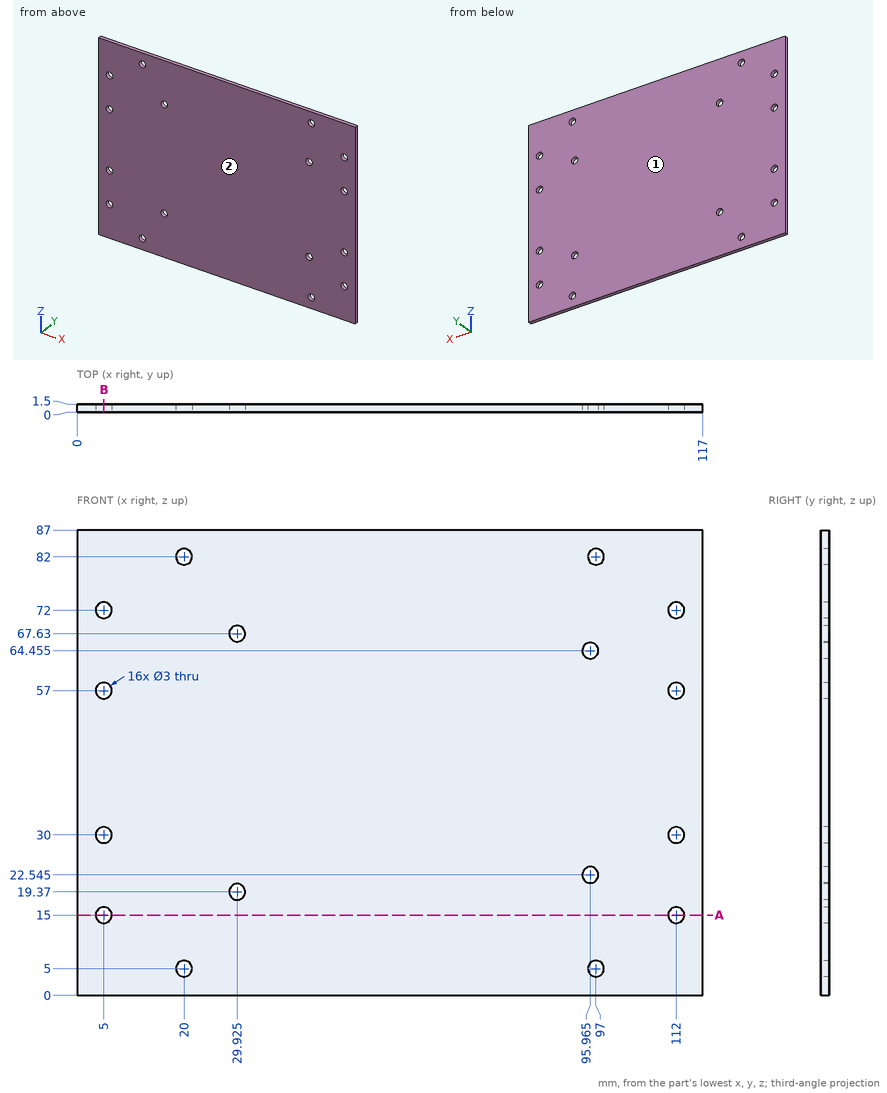
The figure shows three views and two pictorial views of one solid part (mm, origin at its lowest corner). Answer the questions. Give positions to 0.01 mm unless a question says otherwise; leave off trailing zeros. Order: outer loops, then holes, each group sorted by start corner. A loop starts at its lowest first (then second) coordinate and runs counter-clockwise, first axis right, second up. Notation, with made-up numbers: (81, -35) -> (116, -35) arc R8 ccw to (116, -28) -> close; hole circle Ø2 at (15.5, -4). An arc over 180 degrees is marked (long way). One line per item, written item: value.
1) Find the intervals of material crossed by line 1 (Z direction, x = 20, y = 1.2); line 2 (Z direction, x = 112, y = 0.75); line 3 (X direction, y = 0.55, z = 82), in increasing order.
Reported:
line 1: z = 0 to 3.5, 6.5 to 80.5, 83.5 to 87
line 2: z = 0 to 13.5, 16.5 to 28.5, 31.5 to 55.5, 58.5 to 70.5, 73.5 to 87
line 3: x = 0 to 18.5, 21.5 to 95.5, 98.5 to 117
2) Determine the mould class of the marked faces 1 and 2 for opening direction Y: pulls with the +Y half, pulls with the -Y half, needs draft (parallel to the pull), parting line crosses it, or undercut.
Reported:
face 1: pulls with the +Y half
face 2: pulls with the -Y half
3) Find section B-B, the plane x = 5. Determine the outline of the cut face in (y, z).
Reported:
outline: (0, 0) -> (1.5, 0) -> (1.5, 13.5) -> (0, 13.5) -> close; (0, 16.5) -> (1.5, 16.5) -> (1.5, 28.5) -> (0, 28.5) -> close; (0, 31.5) -> (1.5, 31.5) -> (1.5, 55.5) -> (0, 55.5) -> close; (0, 58.5) -> (1.5, 58.5) -> (1.5, 70.5) -> (0, 70.5) -> close; (0, 73.5) -> (1.5, 73.5) -> (1.5, 87) -> (0, 87) -> close
4) Find section A-A, the plane z = 15. Determine the outline of the cut face in (x, y), plus the area to 4 significant figures.
Reported:
outline: (0, 0) -> (3.5, 0) -> (3.5, 1.5) -> (0, 1.5) -> close; (6.5, 0) -> (110.5, 0) -> (110.5, 1.5) -> (6.5, 1.5) -> close; (113.5, 0) -> (117, 0) -> (117, 1.5) -> (113.5, 1.5) -> close
area: 166.5 mm^2
